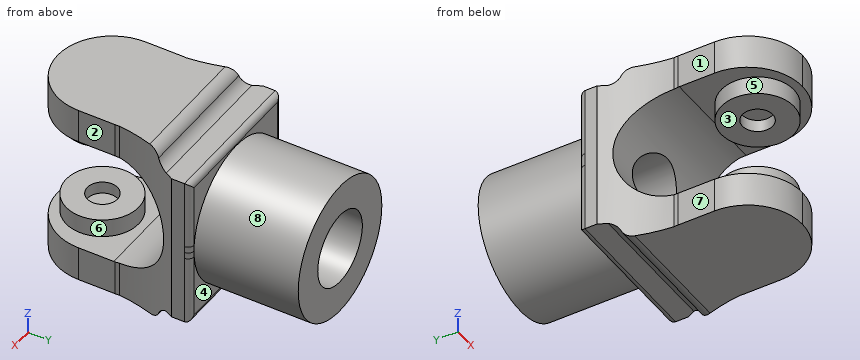
from build123d import *

# Parameters (mm, degrees)
SKETCH1_R           = 14.2875
SKETCH1_R_2         = 7.62
BOSS_EXTRUDE1_DEPTH = 21.844
SKETCH2_W           = 57.929815832
SKETCH2_H           = 52.792019068
BOSS_EXTRUDE2_DEPTH = 37.338
CUT_EXTRUDE2_DEPTH  = 53.792019068
SKETCH5_W           = 10.584509534
SKETCH5_H           = 3.93875565
SKETCH5_W_2         = 10.457509534
CUT_EXTRUDE3_DEPTH  = 37.338
FILLET2_R           = 2.54
SKETCH6_R           = 7.62
CUT_EXTRUDE4_DEPTH  = 37.338
SKETCH7_R           = 7.62
BOSS_EXTRUDE3_DEPTH = 3.81
SKETCH8_R           = 3.175
CUT_EXTRUDE5_DEPTH  = 2.54
FILLET8_R           = 1.27


with BuildPart() as part:
    # Sketch1 → Boss-Extrude1 (new body)
    with BuildSketch(Plane(origin=(0, 0, 0), x_dir=(1, 0, 0), z_dir=(0, 1, 0))):
        Circle(SKETCH1_R)
        Circle(SKETCH1_R_2, mode=Mode.SUBTRACT)
    extrude(amount=BOSS_EXTRUDE1_DEPTH)

    # Sketch2 → Boss-Extrude2 (add)
    with BuildSketch(Plane.XZ):
        Rectangle(SKETCH2_W, SKETCH2_H)
    extrude(amount=BOSS_EXTRUDE2_DEPTH)

    # Sketch4 → Cut-Extrude2 (cut, through all)
    with BuildSketch(Plane.XY.offset(26.396009534)):
        with BuildLine():
            Line((-15.494, -3.81), (-15.494, 0))
            Line((-15.494, 0), (-28.964907916, 0))
            Line((-28.964907916, 0), (-28.964907916, -37.338))
            Line((-28.964907916, -37.338), (0, -37.338))
            ThreePointArc((0, -37.338), (-8.082230509, -33.990230509), (-11.43, -25.908))
            Line((-11.43, -25.908), (-11.43, -18.288))
            ThreePointArc((-11.43, -18.288), (-11.420600472, -17.824551121), (-11.392417347, -17.361864482))
            ThreePointArc((-11.392417347, -17.361864482), (-12.761894788, -10.37972702), (-15.494, -3.81))
        make_face()
        with BuildLine():
            Line((28.964907916, 0), (15.494, 0))
            Line((15.494, 0), (15.494, -3.93875565))
            ThreePointArc((15.494, -3.93875565), (12.774357484, -10.445935023), (11.392417347, -17.361864482))
            ThreePointArc((11.392417347, -17.361864482), (11.420600472, -17.824551121), (11.43, -18.288))
            Line((11.43, -18.288), (11.43, -25.908))
            ThreePointArc((11.43, -25.908), (8.082230509, -33.990230509), (0, -37.338))
            Line((0, -37.338), (28.964907916, -37.338))
            Line((28.964907916, -37.338), (28.964907916, 0))
        make_face()
    extrude(amount=-CUT_EXTRUDE2_DEPTH, mode=Mode.SUBTRACT)

    # Sketch5 → Cut-Extrude3 (cut)
    with BuildSketch(Plane(origin=(15.494, 0, 0), x_dir=(0, 0, -1), z_dir=(1, 0, 0))):
        with BuildLine():
            Line((-15.8115, -5.588), (-15.8115, -3.93875565))
            Line((-15.8115, -3.93875565), (-26.396009534, -3.93875565))
            Line((-26.396009534, -3.93875565), (-26.396009534, -37.338))
            Line((-26.396009534, -37.338), (-19.3675, -37.338))
            Line((-19.3675, -37.338), (-19.3675, -7.9375))
            ThreePointArc((-19.3675, -7.9375), (-17.140553933, -7.44223594), (-15.8115, -5.588))
        make_face()
        with Locations((-21.103754767, -1.969377825)):
            Rectangle(SKETCH5_W, SKETCH5_H)
        with BuildLine():
            Line((-12.192, -18.542), (-12.192, -37.338))
            Line((-12.192, -37.338), (12.192, -37.338))
            Line((12.192, -37.338), (12.192, -18.542))
            ThreePointArc((12.192, -18.542), (0, -6.35), (-12.192, -18.542))
        make_face()
        with Locations((21.167254767, -1.969377825)):
            Rectangle(SKETCH5_W_2, SKETCH5_H)
        with BuildLine():
            Line((26.396009534, -3.93875565), (15.9385, -3.93875565))
            Line((15.9385, -3.93875565), (15.9385, -5.588))
            ThreePointArc((15.9385, -5.588), (17.286672159, -7.413300245), (19.4945, -7.9375))
            Line((19.4945, -7.9375), (19.4945, -37.338))
            Line((19.4945, -37.338), (26.396009534, -37.338))
            Line((26.396009534, -37.338), (26.396009534, -3.93875565))
        make_face()
    extrude(amount=-CUT_EXTRUDE3_DEPTH, mode=Mode.SUBTRACT)

    # Fillet2
    fillet2_edges = [part.edges().sort_by_distance(p)[0] for p in [
        (0.02275558, -7.9375, 19.3675),
        (0.02275558, -7.9375, -19.4945),
    ]]
    fillet(fillet2_edges, radius=FILLET2_R)

    # Sketch6 → Cut-Extrude4 (cut)
    with BuildSketch(Plane(origin=(0, 0, 0), x_dir=(1, 0, 0), z_dir=(0, 1, 0))):
        Circle(SKETCH6_R)
    extrude(amount=-CUT_EXTRUDE4_DEPTH, mode=Mode.SUBTRACT)

    # Sketch7 → Boss-Extrude3 (add)
    with BuildSketch(Plane(origin=(0, 0, 12.192), x_dir=(-1, 0, 0), z_dir=(0, 0, -1))):
        with Locations((0, -27.94)):
            Circle(SKETCH7_R)
    boss_extrude3 = extrude(amount=BOSS_EXTRUDE3_DEPTH)

    # Mirror1: Boss-Extrude3 across plane
    add(boss_extrude3.mirror(Plane.XY))

    # Sketch8 → Cut-Extrude5 (cut)
    with BuildSketch(Plane(origin=(0, 0, 8.382), x_dir=(-1, 0, 0), z_dir=(0, 0, -1))):
        with Locations((0, -27.94)):
            Circle(SKETCH8_R)
    cut_extrude5 = extrude(amount=-CUT_EXTRUDE5_DEPTH, mode=Mode.SUBTRACT)

    # Mirror2: Cut-Extrude5 across plane
    add(cut_extrude5.mirror(Plane.XY), mode=Mode.SUBTRACT)

    # Fillet8
    fillet8_edges = [part.edges().sort_by_distance(p)[0] for p in [
        (0, 0, 15.8115),
        (0, 0, -15.9385),
        (15.494, 0, -0.0635),
        (-15.494, 0, -0.0635),
    ]]
    fillet(fillet8_edges, radius=FILLET8_R)


solid = part.part
Build history of the part. All positions in model axes, mm. Face numbers are marked on the shaded views. A direction names the side the tool comes from. Round coordinates to 2 decimals unless told otherwise and drop trailing zeros. Write each loop counter-clockwise with the first axis right and the second up, starting at its lowest first coordinate (ties: lowest second). Pieces come first, ordered by that corner, then holes. Notation, with made-up numbers: M 63,-26.5 L 116,-26.5 A18 cw 116,-13.5 Z; hole C -20.75,82 d3. An arc over 180 degrees is marked long. Answer in a Markdown table with one row per item.
1. Saw through at C-C (z = -6). List the corners of the cut face in (x, y).
Geometry check:
| item | result |
|---|---|
| outline | M -15.49,-3.81 A35.56 cw -13.6,-7.93 L -4.7,-7.93 L -4.7,21.84 L -12.97,21.84 L -12.97,0 L -14.22,0 A1.27 ccw -15.49,-1.27 Z; M 4.7,-7.93 L 13.65,-7.93 A35.56 cw 15.49,-3.94 L 15.49,-1.27 A1.27 ccw 14.22,0 L 12.97,0 L 12.97,21.84 L 4.7,21.84 Z |
2. Probe L1, parallel to Z at x = 0, y = -2.5; L2, parallel to Z at x = 0, y = 11.75. List the from-to ranges inside material, lowest first. Write a range as [from, to].
Geometry check:
| item | result |
|---|---|
| L1 | [-15.94, -7.62], [7.62, 15.81] |
| L2 | [-14.29, -7.62], [7.62, 14.29] |
3. Flat gauge pins, fed straight in: P1, Ø1, axis at x = -12, y = 13.5, coming from the +Z side; P2, Ø8, axis at y = -21, z = -15, coming from the +X side; P3, Ø3, axis at x = -2.5, z = -13.5, coming from the -Y side. Where does each tip first touch, or does it go through?
Geometry check:
| item | result |
|---|---|
| P1 | z = 8.48 |
| P2 | x = 11.43 |
| P3 | y = -37.29 |
4. Which spindle directions (+Z, -Z, +X, -X, +Y, -Y) get a long thin tool onto all of the face, cutting with end or side? Do the marked faces 1, 2, 3, 4 and 5. Say none if no direction does.
Geometry check:
| item | result |
|---|---|
| face 1 | +Z, -Z, -X, -Y |
| face 2 | +Z, -Z, +X, -Y |
| face 3 | +X, -X, -Y |
| face 4 | -Z, +Y |
| face 5 | none |
5. Mould opens along Z. For the marked faces 6, 7 and 8 say: +Z half, -Z half, draft (parallel to the pull), parting line (faces both ways), or undercut.
Geometry check:
| item | result |
|---|---|
| face 6 | undercut |
| face 7 | draft |
| face 8 | parting line |
6. Saw through at A-A (z = 9.5). List the corners of the cut face in (x, y) (3 decimals).
Geometry check:
| item | result |
|---|---|
| outline | M -15.494,-3.81 A35.56 cw -12.609,-10.9 L 12.639,-10.9 A35.56 cw 15.494,-3.939 L 15.494,-1.27 A1.27 ccw 14.224,0 L 10.672,0 L 10.672,21.844 L -10.672,21.844 L -10.672,0 L -14.224,0 A1.27 ccw -15.494,-1.27 Z; C 0,-27.94 d15.24; hole C 0,-27.94 d6.35 |
7. Saw through at D-D (y = -16). List the corners of the cut face in (x, z), and give its area (3 significant figures).
Geometry check:
| item | result |
|---|---|
| outline | M -11.55,-19.49 L 11.55,-19.49 L 11.55,-11.92 L -11.55,-11.92 Z; M -11.55,11.92 L 11.55,11.92 L 11.55,19.37 L -11.55,19.37 Z |
| area | 347 mm2 |
